For this review, use the dimensioned drawing (mm, ordinates from the lowest corner) and the shaded views. Round coordinates to 2 decimals unless told otherwise and drop trailing zeros. Order: outer loops, then holes, each group sorted by start corner. A loop starts at its lowest first (then second) coordinate and runs counter-clockwise, first axis right, second up. Notation, with made-up numbers: (-7.5, -33) -> (-3.5, -33) arc R15 ccw to (-3.5, -22) -> close; hole circle Ø9 at (32, 56). An arc over 180 degrees is marked (long way). Answer in a Markdown table with one row per item.
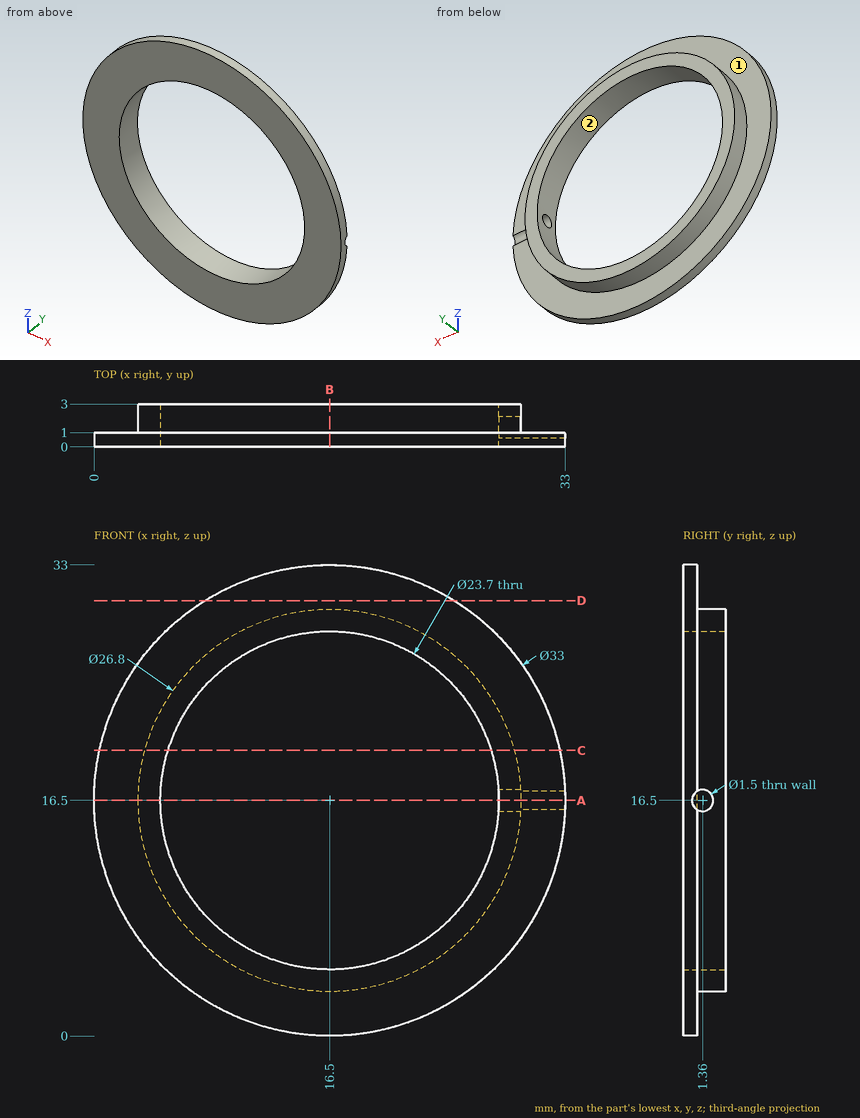
Q1. The part is to be moulded in two halves that separate along X. For the marked faces 1 and 2, say which applies: +X half, -X half, draft (parallel to the pull), parting line (faces both ways), or undercut.
Answer key:
| item | result |
|---|---|
| face 1 | draft |
| face 2 | undercut |
Q2. Take a section at C-C, the plane z = 20. Write out the cut boundary in (x, y).
Answer key:
| item | result |
|---|---|
| outline | (0.38, 0) -> (5.18, 0) -> (5.18, 3) -> (3.57, 3) -> (3.57, 1) -> (0.38, 1) -> close; (27.82, 0) -> (32.62, 0) -> (32.62, 1) -> (29.43, 1) -> (29.43, 3) -> (27.82, 3) -> close |
Q3. To check wall thickness, follow probe 1 along Z at (x, y) = (16.5, 2.25); probe 2 along X at (y, z) = (2.5, 15.5); probe 3 along Z at (x, y) = (10, 2.25). State the ranges of each line that lie inside material, in increasing order.
Answer key:
| item | result |
|---|---|
| probe 1 | z = 3.1 to 4.65, 28.35 to 29.9 |
| probe 2 | x = 3.14 to 4.69, 28.31 to 29.86 |
| probe 3 | z = 4.78 to 6.59, 26.41 to 28.22 |
Q4. Take a section at D-D, the plane z = 30.5. Write out the cut boundary in (x, y).
Answer key:
| item | result |
|---|---|
| outline | (7.77, 0) -> (25.23, 0) -> (25.23, 1) -> (7.77, 1) -> close |
Q5. Clearance check with flat-ended pins moving along their axes: pin 1 Ø1.7 at (y, z) = (1.36, 16.5) entering from -X; pin 2 Ø12 at (x, z) = (14, 21) entering from +Y; pin 3 Ø1.5 at (y, z) = (2.5, 7.5) entering from -X. State where each tip first meets the part, or that it passes through.
Answer key:
| item | result |
|---|---|
| pin 1 | stops at x = 0 |
| pin 2 | passes through |
| pin 3 | stops at x = 5.94 |
Q6. Take a section at A-A, the plane z = 16.5. Write out the cut boundary in (x, y).
Answer key:
| item | result |
|---|---|
| outline | (0, 0) -> (4.65, 0) -> (4.65, 3) -> (3.1, 3) -> (3.1, 1) -> (0, 1) -> close; (28.35, 0) -> (33, 0) -> (33, 0.61) -> (28.35, 0.61) -> close; (28.35, 2.11) -> (29.9, 2.11) -> (29.9, 3) -> (28.35, 3) -> close |
Q7. Take a section at B-B, the plane x = 16.5. Write out the cut boundary in (y, z), then the cut area to 3 significant figures.
Answer key:
| item | result |
|---|---|
| outline | (0, 0) -> (1, 0) -> (1, 3.1) -> (3, 3.1) -> (3, 4.65) -> (0, 4.65) -> close; (0, 28.35) -> (3, 28.35) -> (3, 29.9) -> (1, 29.9) -> (1, 33) -> (0, 33) -> close |
| area | 15.5 mm^2 |
